from build123d import *

# Parameters (mm, degrees)
CHAMFER1_SIZE           = 0.762
SKETCH5_W               = 6.35
SKETCH5_H               = 0.7874
CUT_EXTRUDE1_DEPTH      = 10.4488
CUT_EXTRUDE1_DEPTH_BACK = 10.4488
SKETCH6_W               = 6.35
SKETCH6_H               = 0.7874
CUT_EXTRUDE2_DEPTH      = 10.4488
CUT_EXTRUDE2_DEPTH_BACK = 10.4488


with BuildPart() as part:
    # Sketch1 → Revolve1 (revolve)
    with BuildSketch(Plane(origin=(0, 0, 0), x_dir=(-1, 0, 0), z_dir=(0, 0, -1)), mode=Mode.PRIVATE) as revolve1_sk:
        with BuildLine():
            Line((-99.4156, 2.786922533), (-99.4156, 0))
            Line((-99.4156, 0), (0, 0))
            Line((0, 0), (0, 9.4488))
            Line((0, 9.4488), (-81.7626, 9.4488))
            Line((-81.7626, 9.4488), (-81.7626, 3.175))
            Line((-81.7626, 3.175), (-98.3996, 3.175))
            ThreePointArc((-98.3996, 3.175), (-98.943396865, 3.074678675), (-99.4156, 2.786922533))
        make_face()
    revolve(revolve1_sk.sketch.rotate(Axis((99.4156, 0, 0), (-1, 0, 0)), 270), axis=Axis((99.4156, 0, 0), (-1, 0, 0)))  # turned: the seam where the file's is

    # Sketch2 → Cut-Revolve1 (revolve, cut)
    with BuildSketch(Plane(origin=(0, 0, 0), x_dir=(-1, 0, 0), z_dir=(0, 0, -1)), mode=Mode.PRIVATE) as cut_revolve1_sk:
        Polygon((-13.97, 4.9784), (-13.97, 0), (0, 0), (0, 6.1849), (-2.5527, 5.642306865), (-3.216606865, 4.9784), align=None)
    revolve(cut_revolve1_sk.sketch.rotate(Axis((13.97, 0, 0), (-1, 0, 0)), 270), axis=Axis((13.97, 0, 0), (-1, 0, 0)), mode=Mode.SUBTRACT)  # turned: the seam where the file's is

    # Sketch3 → Cut-Revolve2 (revolve, cut)
    with BuildSketch(Plane(origin=(0, 0, 0), x_dir=(-1, 0, 0), z_dir=(0, 0, -1)), mode=Mode.PRIVATE) as cut_revolve2_sk:
        Polygon((-99.4156, 1.7272), (-99.4156, 0), (-93.0656, 0), (-94.103406461, 1.7272), align=None)
    revolve(cut_revolve2_sk.sketch.rotate(Axis((66.313858967, 0, 0), (-1, 0, 0)), 270), axis=Axis((66.313858967, 0, 0), (-1, 0, 0)), mode=Mode.SUBTRACT)  # turned: the seam where the file's is

    # Chamfer1
    chamfer1_edges = [part.edges().sort_by_distance(p)[0] for p in [
        (81.7626, 0, -9.4488),
        (0, 0, -9.4488),
    ]]
    chamfer(chamfer1_edges, length=CHAMFER1_SIZE)

    # Sketch5 → Cut-Extrude1 (cut, two sides)
    with BuildSketch(Plane(origin=(0, 0, 0), x_dir=(1, 0, 0), z_dir=(0, 1, 0))) as cut_extrude1_sk:
        with Locations((3.175, 9.0551)):
            Rectangle(SKETCH5_W, SKETCH5_H)
        with Locations((3.175, -9.0551)):
            Rectangle(SKETCH5_W, SKETCH5_H)
    extrude(amount=CUT_EXTRUDE1_DEPTH, mode=Mode.SUBTRACT)
    extrude(cut_extrude1_sk.sketch, amount=-CUT_EXTRUDE1_DEPTH_BACK, mode=Mode.SUBTRACT)

    # Sketch6 → Cut-Extrude2 (cut, two sides)
    with BuildSketch(Plane(origin=(0, 0, 0), x_dir=(1, 0, 0), z_dir=(0, 1, 0))) as cut_extrude2_sk:
        with Locations((78.5876, 9.0551)):
            Rectangle(SKETCH6_W, SKETCH6_H)
        with Locations((78.5876, -9.0551)):
            Rectangle(SKETCH6_W, SKETCH6_H)
    extrude(amount=CUT_EXTRUDE2_DEPTH, mode=Mode.SUBTRACT)
    extrude(cut_extrude2_sk.sketch, amount=-CUT_EXTRUDE2_DEPTH_BACK, mode=Mode.SUBTRACT)


solid = part.part
Can you work these out from the model? Positions are in its coordinate system, mm. A direction names the side the tool comes from. Give positions to 0.01 mm unless a question says otherwise; leave off trailing zeros. Write each loop counter-clockwise with the first axis right and the second up, starting at its lowest first coordinate (ties: lowest second). Pieces come first, ordered by that corner, then holes. Notation, with made-up numbers: M 8,-11.75 L 65,-11.75 A21 ccw 65,10.25 Z; hole C 15.5,71 d7. An arc over 180 degrees is marked long. Answer in a Markdown table with one row per item. Add a question column.
Item 1: On a 3-axis mill with a long thin cutter (end or side, diameter ignored), from which of +Z, -Z, +X, -X, +Y, -Y can I reach the whole of each face in a straight line? I mean faces 1 (the flat face through (3, 0, 8.661)), 2 (the flat face through (13.97, 0, 0)), 3 (the cylindrical face through (96.797, -1.686, -0.374)). Say none if no direction works.
Item 2: For pin 1 Ø1.9 at (x, y) = (3.5, 0) entering from +Z; pin 2 Ø1 at (x, y) = (34.5, 4.5) entering from +Z; pin 3 Ø7 at (x, y) = (3, 1.5) entering from -Z; pin 4 Ø8 at (x, z) = (43, 0.5) entering from +Y, each with a flat end and sliding along its axis, tell me the tip position at first contact or that it passes through.
Item 3: Imagine slicing it at A-A, the plane x = 47.5. Write out the boundary of the cut face in (y, z), plus the area to 3 significant figures.
Item 4: We'd pull the mould along Z, two halves only. Please class faces 4 (the flat face through (99.416, -2, 0)), 5 (the conical face through (81.63, -8.82, -0.18)), 6 (the cylindrical face through (8.669, 1.495, 4.749)): released by +Z, released by -Z, zero draft, split by the parting line, or undercut.
Item 5: Please list where these lines run through material, in increasing order: L1, parallel to Y at x = 97.35, z = 0 (3 decimals); L2, parallel to X at y = 1.75, z = -1; L3, parallel to X at y = -1, z = -6.25.
Evaluation:
| question | item | result |
|---|---|---|
| 1 | face 1 | +Z, -X, +Y, -Y |
| 1 | face 2 | -X |
| 1 | face 3 | +X |
| 2 | pin 1 | stops at z = 8.66 |
| 2 | pin 2 | stops at z = 8.56 |
| 2 | pin 3 | stops at z = -9.44 |
| 2 | pin 4 | stops at y = 9.45 |
| 3 | outline | C 0,0 d18.9 |
| 3 | area | 280 mm² |
| 4 | face 4 | zero draft |
| 4 | face 5 | split by the parting line |
| 4 | face 6 | undercut |
| 5 | L1 | y = -3.175 to -1.727, 1.727 to 3.175 |
| 5 | L2 | x = 13.97 to 99.42 |
| 5 | L3 | x = 0 to 81.76 |
